```python
from build123d import *

# Parameters (mm, degrees)
BASE_FLANGE1_DEPTH                 = 10
F_3_0MM_TRANSITIONAL_DOWEL_HOLE1_D = 3
F_3_0MM_PRESS_DOWEL_HOLE1_D        = 3


# Sheet-metal steps are written as plain solids
with BuildPart() as part:
    # Sketch1 → Base-Flange1 (new body)
    with BuildSketch(Plane(origin=(0, 0, 0), x_dir=(1, 0, 0), z_dir=(0, 1, 0))):
        with BuildLine():
            Line((0, 0), (0, -19.2634))
            ThreePointArc((0, -19.2634), (0.215745145, -19.784254855), (0.7366, -20))
            Line((0.7366, -20), (20, -20))
            Line((20, -20), (20, -21.5))
            Line((20, -21.5), (0.7366, -21.5))
            ThreePointArc((0.7366, -21.5), (-0.844915027, -20.844915027), (-1.5, -19.2634))
            Line((-1.5, -19.2634), (-1.5, 0))
            Line((-1.5, 0), (0, 0))
        make_face()
    extrude(amount=BASE_FLANGE1_DEPTH)

    # Ø3.0mm Transitional Dowel Hole1 (through all)
    with Locations(Plane.ZY.offset(1.5)):
        with Locations((16.387023366, 4.560762846), (6.466703516, 4.560762846)):
            Hole(F_3_0MM_TRANSITIONAL_DOWEL_HOLE1_D / 2)

    # Ø3.0mm Press Dowel Hole1 (through all)
    with Locations(Plane(origin=(0, 0, 20), x_dir=(-1, 0, 0), z_dir=(0, 0, -1))):
        with Locations((-4.7366, 5), (-16, 5)):
            Hole(F_3_0MM_PRESS_DOWEL_HOLE1_D / 2)


solid = part.part
```
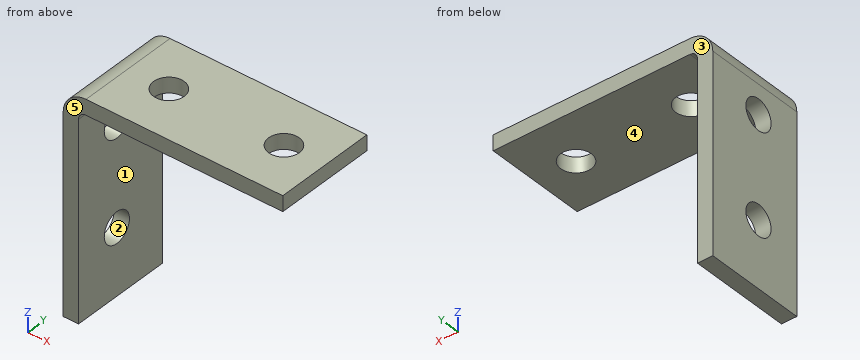
CAD build for the part. Positions are in the model's coordinates, mm. Face numbers are marked on the shaded views. A direction names the side the tool comes from. Coordinates: 2 decimals unless noted, no trailing zeros. Loops run counter-clockwise (first coordinate to the right, second up) from the corner with the lowest first, then second, coordinate; pieces in that order, holes last. Notation, with made-up numbers: (-15, 25) - (29, 25) arc R13 cw to (29, 45) - close; hole circle Ø1 at (65.25, -24.75). An arc over 180 degrees is marked (long way). Use CSV: the item, a comma, the result in double quotes. Start each with the question number.
Q1. Cut at A-A, the plane x = 16. List the corners of the cut face in (y, z).
Q2. Probe probe 1 along Y at (x, z) = (16, 20.25); probe 2 along X at (y, z) = (2.75, 13.75); probe 3 along Z at (x, y) = (6.25, 8.25). List the from-to ranges inside material, lowest first. Write a range as from..to.
Q3. Cut at C-C, the plane z = 5.75. List the corners of the cut face in (x, y), then the cut area to 3 significant figures.
Q4. Cut at D-D, the plane x = 1.5. List the corners of the cut face in (y, z), then the cut area to 3 significant figures.
Q5. Cut at B-B, the plane y = 5.75. List the corners of the cut face in (x, z).
Q6. Drop flat-ended pins along their axis: P1, Ø2, axis at y = 7.5, z = 5, coming from the +X side; P2, Ø3, axis at x = 16, y = 6.5, coming from the -Z side. Give the stop position or say it passes through.
Q7. 3-axis set-ups, long thin cutter, end or side, ignore diameter. For the marked faces 4 and 5: which of +Z, -Z, +X, -X, +Y, -Y reach the whole face in a straight line?
Q8. Two-plate mould, pull along Y, no slides. Class the marked faces 1, 2 and 3: +Y half, -Y half, draft (parallel to the pull), parting line (faces both ways), or undercut.
Here are the results:
1,outline,"(0, 20) - (3.5, 20) - (3.5, 21.5) - (0, 21.5) - close; (6.5, 20) - (10, 20) - (10, 21.5) - (6.5, 21.5) - close"
2,probe 1,"0..3.5, 6.5..10"
2,probe 2,"-1.5..0"
2,probe 3,"20..21.5"
3,outline,"(-1.5, 0) - (0, 0) - (0, 3.24) - (-1.5, 3.24) - close; (-1.5, 5.88) - (0, 5.88) - (0, 10) - (-1.5, 10) - close"
3,area,"11.0 mm2"
4,outline,"(0, 20) - (10, 20) - (10, 21.5) - (0, 21.5) - close"
4,area,"15.0 mm2"
5,outline,"(-1.5, 0) - (0, 0) - (0, 5.55) - (-1.5, 5.55) - close; (-1.5, 7.38) - (0, 7.38) - (0, 15.47) - (-1.5, 15.47) - close; (-1.5, 17.3) - (0, 17.3) - (0, 19.26) arc R0.74 cw to (0.74, 20) - (3.44, 20) - (3.44, 21.5) - (0.74, 21.5) arc R2.24 ccw to (-1.5, 19.26) - close; (6.04, 20) - (14.7, 20) - (14.7, 21.5) - (6.04, 21.5) - close; (17.3, 20) - (20, 20) - (20, 21.5) - (17.3, 21.5) - close"
6,P1,"x = 0"
6,P2,"z = 20"
7,face 4,"-Z, +X, +Y, -Y"
7,face 5,"+Z, -Z, +X, -X, -Y"
8,face 1,"draft"
8,face 2,"undercut"
8,face 3,"+Y half"
